Check sheet for the modelled part. Datum: model origin and axes. Units: mm. Round coordinates to 2 decimals unless told otherwise and drop trailing zeros. Write each loop counter-clockwise with the first axis right and the second up, starting at its lowest first coordinate (ties: lowest second). Pieces come first, ordered by that corner, then holes.
from build123d import *

# Parameters (mm, degrees)
SKETCH1_W           = 95
SKETCH1_H           = 73.7
BOSS_EXTRUDE1_DEPTH = 5
CUT_EXTRUDE1_REACH  = 7
SKETCH2_W           = 5.4
SKETCH2_H           = 8.6
CUT_EXTRUDE2_REACH  = 7


with BuildPart() as part:
    # Sketch1 → Boss-Extrude1 (new body)
    with BuildSketch(Plane(origin=(0, 0, 0), x_dir=(1, 0, 0), z_dir=(0, 1, 0))):
        with Locations((3.050458716, -12.337385321)):
            Rectangle(SKETCH1_W, SKETCH1_H)
    extrude(amount=BOSS_EXTRUDE1_DEPTH)

    # Sketch2 → Cut-Extrude1 (cut, up to next)
    with BuildSketch(Plane(origin=(0, 5, 0), x_dir=(1, 0, 0), z_dir=(0, 1, 0)), mode=Mode.PRIVATE) as cut_extrude1_sk1:
        with Locations((-41.749541284, 6.712614679)):
            Rectangle(SKETCH2_W, SKETCH2_H)
    cut_extrude1_tool1 = extrude(cut_extrude1_sk1.sketch, amount=-CUT_EXTRUDE1_REACH, mode=Mode.PRIVATE) & part.part
    add(cut_extrude1_tool1.solids().sort_by_distance((-41.749541, 5, -6.712615))[0], mode=Mode.SUBTRACT)
    # Sketch2 → Cut-Extrude1 (cut, up to next)
    with BuildSketch(Plane(origin=(0, 5, 0), x_dir=(1, 0, 0), z_dir=(0, 1, 0)), mode=Mode.PRIVATE) as cut_extrude1_sk2:
        with Locations((-41.749541284, -27.687385321)):
            Rectangle(SKETCH2_W, SKETCH2_H)
    cut_extrude1_tool2 = extrude(cut_extrude1_sk2.sketch, amount=-CUT_EXTRUDE1_REACH, mode=Mode.PRIVATE) & part.part
    add(cut_extrude1_tool2.solids().sort_by_distance((-41.749541, 5, 27.687385))[0], mode=Mode.SUBTRACT)
    # Sketch2 → Cut-Extrude1 (cut, up to next)
    with BuildSketch(Plane(origin=(0, 5, 0), x_dir=(1, 0, 0), z_dir=(0, 1, 0)), mode=Mode.PRIVATE) as cut_extrude1_sk3:
        with Locations((47.850458716, 6.712614679)):
            Rectangle(SKETCH2_W, SKETCH2_H)
    cut_extrude1_tool3 = extrude(cut_extrude1_sk3.sketch, amount=-CUT_EXTRUDE1_REACH, mode=Mode.PRIVATE) & part.part
    add(cut_extrude1_tool3.solids().sort_by_distance((47.850459, 5, -6.712615))[0], mode=Mode.SUBTRACT)
    # Sketch2 → Cut-Extrude1 (cut, up to next)
    with BuildSketch(Plane(origin=(0, 5, 0), x_dir=(1, 0, 0), z_dir=(0, 1, 0)), mode=Mode.PRIVATE) as cut_extrude1_sk4:
        with Locations((47.850458716, -27.687385321)):
            Rectangle(SKETCH2_W, SKETCH2_H)
    cut_extrude1_tool4 = extrude(cut_extrude1_sk4.sketch, amount=-CUT_EXTRUDE1_REACH, mode=Mode.PRIVATE) & part.part
    add(cut_extrude1_tool4.solids().sort_by_distance((47.850459, 5, 27.687385))[0], mode=Mode.SUBTRACT)

    # Sketch3 → Cut-Extrude2 (cut, up to next)
    with BuildSketch(Plane(origin=(0, 5, 0), x_dir=(1, 0, 0), z_dir=(0, 1, 0)), mode=Mode.PRIVATE) as cut_extrude2_sk1:
        with BuildLine():
            Line((-3.185639247, -3.188538713), (-3.185639247, -23.188538713))
            ThreePointArc((-3.185639247, -23.188538713), (-15.685639247, -35.688538713), (-28.185639247, -23.188538713))
            Line((-28.185639247, -23.188538713), (-28.185639247, -3.188538713))
            ThreePointArc((-28.185639247, -3.188538713), (-15.685639247, 9.311461287), (-3.185639247, -3.188538713))
        make_face()
    cut_extrude2_tool1 = extrude(cut_extrude2_sk1.sketch, amount=-CUT_EXTRUDE2_REACH, mode=Mode.PRIVATE) & part.part
    add(cut_extrude2_tool1.solids().sort_by_distance((-15.685639, 5, 13.188539))[0], mode=Mode.SUBTRACT)


solid = part.part
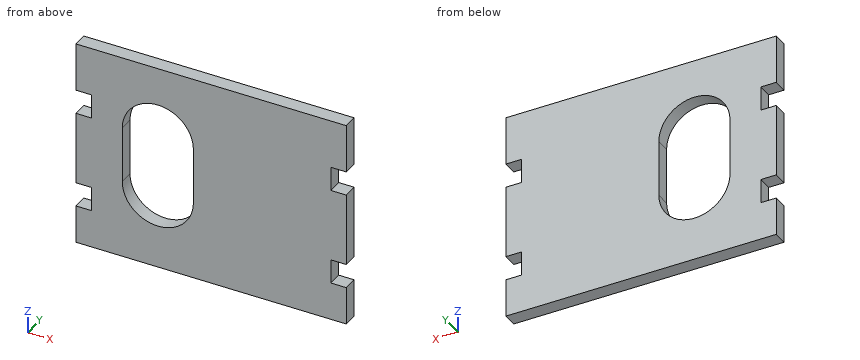
1. Sectioned sample at B-B, the plane x = -27. Enter the section's corners in (y, z).
2. Go/stop test with flat-tipped pins: pin 1 (2 mm diameter, centred on y = 3, z = -4, fed in from +X); pin 2 (1.5 mm diameter, centred on y = 1.5, z = -5.5, fed in from -X). Record where each tip stops, or that it passes through.
3. Scan lines: line 1 along Z through (x, y) = (45.5, 1.7); line 2 along X through (y, z) = (0.3, 10); line 3 along Z through (x, y) = (-18.5, 2.4). Record each from-to range of solid material in increasing order.
4. Sectioned sample at A-A, the plane z = 19. Enter the section's corners in (x, y).
5. Sectioned sample at C-C, the plane y = 2.1. Enter the section's corners in (x, z), plus the area to 3 significant figures.
Computed values:
1. outline: (0, -24.51) - (5, -24.51) - (5, -2.13) - (0, -2.13) - close; (0, 28.5) - (5, 28.5) - (5, 49.19) - (0, 49.19) - close
2. pin 1: stops at x = 45.15
2. pin 2: stops at x = -39.05
3. line 1: z = -24.51 to -11.01, -2.41 to 23.39, 31.99 to 49.19
3. line 2: x = -44.45 to -28.19, -3.19 to 50.55
3. line 3: z = -24.51 to -8.99, 35.37 to 49.19
4. outline: (-44.45, 0) - (-28.19, 0) - (-28.19, 5) - (-44.45, 5) - close; (-3.19, 0) - (50.55, 0) - (50.55, 5) - (-3.19, 5) - close
5. outline: (-44.45, -24.51) - (50.55, -24.51) - (50.55, -11.01) - (45.15, -11.01) - (45.15, -2.41) - (50.55, -2.41) - (50.55, 23.39) - (45.15, 23.39) - (45.15, 31.99) - (50.55, 31.99) - (50.55, 49.19) - (-44.45, 49.19) - (-44.45, 31.99) - (-39.05, 31.99) - (-39.05, 23.39) - (-44.45, 23.39) - (-44.45, -2.41) - (-39.05, -2.41) - (-39.05, -11.01) - (-44.45, -11.01) - close; hole (-28.19, 3.19) arc R12.5 ccw to (-3.19, 3.19) - (-3.19, 23.19) arc R12.5 ccw to (-28.19, 23.19) - close
5. area: 5,820 mm2
